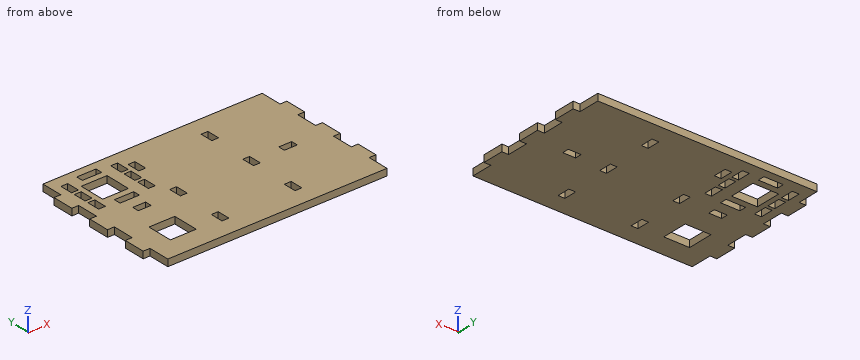
```python
from build123d import *

# Parameters (mm, degrees)
SKETCH1_W           = 6
SKETCH1_H           = 3.125
SKETCH1_W_2         = 3.175
SKETCH1_H_2         = 6
BOSS_EXTRUDE1_DEPTH = 1.5875


with BuildPart() as part:
    # Sketch1 → Boss-Extrude1 (new body, symmetric)
    with BuildSketch(Plane.XY):
        Polygon((54.175, 0), (54.175, 5), (51, 5), (51, 15), (54.175, 15), (54.175, 25), (51, 25), (51, 35), (17, 35), (0, 35), (-17, 35), (-51, 35), (-51, 25), (-54.175, 25), (-54.175, 15), (-51, 15), (-51, 5), (-54.175, 5), (-54.175, -5), (-51, -5), (-51, -15), (-54.175, -15), (-54.175, -25), (-51, -25), (-51, -35), (0, -35), (51, -35), (51, -25), (54.175, -25), (54.175, -15), (51, -15), (51, -5), (54.175, -5), align=None)
        Polygon((-41.5, -13), (-34, -13), (-29.5, -13), (-29.5, -25), (-34, -25), (-41.5, -25), align=None, mode=Mode.SUBTRACT)
        Polygon((-18.5875, -23.333333333), (-18.5875, -20.333333333), (-15.4125, -20.333333333), (-15.4125, -26.333333333), (-18.5875, -26.333333333), align=None, mode=Mode.SUBTRACT)
        Polygon((18.5875, -20.333333333), (18.5875, -23.333333333), (18.5875, -26.333333333), (15.4125, -26.333333333), (15.4125, -20.333333333), align=None, mode=Mode.SUBTRACT)
        with Locations((-34, 0)):
            Rectangle(SKETCH1_W, SKETCH1_H, mode=Mode.SUBTRACT)
        Polygon((-38.5, 6.825), (-38.5, 10), (-34, 10), (-29.5, 10), (-29.5, 6.825), align=None, mode=Mode.SUBTRACT)
        Polygon((-47.175, 14.4125), (-45.5875, 14.4125), (-44, 14.4125), (-44, 8.4125), (-47.175, 8.4125), align=None, mode=Mode.SUBTRACT)
        with Locations((-17, 0)):
            Rectangle(SKETCH1_W_2, SKETCH1_H_2, mode=Mode.SUBTRACT)
        Polygon((-24, 14.4125), (-22.4125, 14.4125), (-20.825, 14.4125), (-20.825, 8.4125), (-24, 8.4125), align=None, mode=Mode.SUBTRACT)
        Polygon((-44, 22), (-44, 19), (-44, 16), (-45.5875, 16), (-47.175, 16), (-47.175, 22), (-45.5875, 22), align=None, mode=Mode.SUBTRACT)
        Polygon((-41.5, 25), (-34, 25), (-29.5, 25), (-29.5, 13), (-34, 13), (-41.5, 13), align=None, mode=Mode.SUBTRACT)
        Polygon((-44, 23.5875), (-45.5875, 23.5875), (-47.175, 23.5875), (-47.175, 29.5875), (-44, 29.5875), align=None, mode=Mode.SUBTRACT)
        Polygon((-38.5, 31.175), (-29.5, 31.175), (-29.5, 28), (-34, 28), (-38.5, 28), align=None, mode=Mode.SUBTRACT)
        Polygon((-20.825, 16), (-22.4125, 16), (-24, 16), (-24, 19), (-24, 22), (-22.4125, 22), (-20.825, 22), align=None, mode=Mode.SUBTRACT)
        Polygon((-18.5875, 20.333333333), (-18.5875, 23.333333333), (-18.5875, 26.333333333), (-15.4125, 26.333333333), (-15.4125, 20.333333333), align=None, mode=Mode.SUBTRACT)
        Polygon((-20.825, 23.5875), (-22.4125, 23.5875), (-24, 23.5875), (-24, 29.5875), (-20.825, 29.5875), align=None, mode=Mode.SUBTRACT)
        with Locations((17, 0)):
            Rectangle(SKETCH1_W_2, SKETCH1_H_2, mode=Mode.SUBTRACT)
        Polygon((37, 1.5625), (37, 0), (37, -1.5625), (31, -1.5625), (31, 1.5625), align=None, mode=Mode.SUBTRACT)
        Polygon((18.5875, 23.333333333), (18.5875, 20.333333333), (15.4125, 20.333333333), (15.4125, 26.333333333), (18.5875, 26.333333333), align=None, mode=Mode.SUBTRACT)
    extrude(amount=BOSS_EXTRUDE1_DEPTH, both=True)


solid = part.part
```
Read the model definition and answer for the solid it produces. Units are mm, in the model's axes. Give positions to 0.01 mm unless a question says otherwise; leave off trailing zeros. Order: outer loops, then holes, each group sorted by start corner. A loop starts at its lowest first (then second) coordinate and runs counter-clockwise, first axis right, second up. Notation, with made-up numbers: (73, 14.25) -> (111, 14.25) arc R21 cw to (111, 27.25) -> close; hole circle Ø2 at (-34.5, 53.5). An arc over 180 degrees is marked (long way). One line per item, written item: value. Start each with the question number.
(1) The part is cut by section C-C (y = -11). Determine the outline of the cut face in (x, z), and give its area (3 significant figures).
(2) Straight lines are drawn through the part: L1, parallel to X at y = 16.5, z = 1.15 (3 decimals); L2, parallel to Y at x = -44.5, z = 1; L3, parallel to Y at x = -35, z = 0.45 (1 decimal). For each, find the intervals that lie inside material, in ascending order.
(3) The part is cut by section B-B (z = -0.55). State how many separate pieces and enclosed holes the cut face has, and give its area (3 significant figures).
(4) Flat-ended cylindrical pins translate along their axes: P1, Ø1, axis at y = 10.5, z = 0.5, coming from the +X side; P2, Ø1, axis at x = -52.5, z = -0.5, coming from the -Y side; P3, Ø5, axis at x = -39, y = -24.5, coming from the -Z side; P4, Ø1.6, axis at y = -31, z = 0.5, coming from the -X side. Find the tip coordinate at first contact, or state that the pin passes through.
(5) The part is cut by section A-A (y = -23.5). Determine the outline of the cut face in (x, z) (1 decimal).
Taken from the geometry:
1. outline: (-51, -1.59) -> (51, -1.59) -> (51, 1.59) -> (-51, 1.59) -> close
1. area: 324 mm^2
2. L1: -54.175 to -47.175, -44 to -41.5, -29.5 to -24, -20.825 to 54.175
2. L2: -35 to 8.41, 14.41 to 16, 22 to 23.59, 29.59 to 35
2. L3: -35 to -25, -13 to -1.6, 1.6 to 6.8, 10 to 13, 25 to 28, 31.2 to 35
3. separate pieces: 1
3. enclosed holes: 18
3. area: 6,720 mm^2
4. P1: x = 51
4. P2: y = -25
4. P3: z = -1.59
4. P4: x = -51
5. outline: (-54.2, -1.6) -> (-41.5, -1.6) -> (-41.5, 1.6) -> (-54.2, 1.6) -> close; (-29.5, -1.6) -> (-18.6, -1.6) -> (-18.6, 1.6) -> (-29.5, 1.6) -> close; (-15.4, -1.6) -> (15.4, -1.6) -> (15.4, 1.6) -> (-15.4, 1.6) -> close; (18.6, -1.6) -> (54.2, -1.6) -> (54.2, 1.6) -> (18.6, 1.6) -> close
